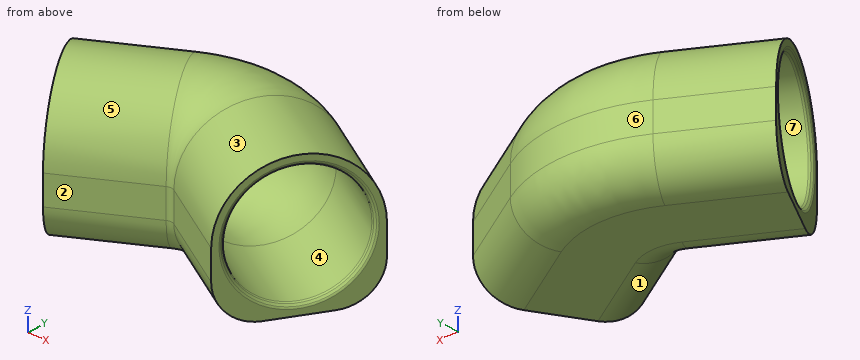
```python
from build123d import *

# Parameters (mm, degrees)
F1_R    = 11.1633
F3_R    = 7.62
F4_SIZE = 0.635
F5_R    = 0.508


with BuildPart() as f2:
    # F2: sweep along a path in F0
    with BuildLine(Plane.XY) as f2_path:
        Line((-21.9970452561, -12.7), (-6.35, -3.6661742094))
        ThreePointArc((-6.35, -3.6661742094), (0, -1.9646968374), (6.35, -3.6661742094))
        Line((6.35, -3.6661742094), (21.9970452561, -12.7))
    # F1 (on Right) → F2 (sweep)
    with BuildSketch(Plane.YZ):
        with BuildLine():
            ThreePointArc((0, -13.1633), (9.3078586928, -9.3078586928), (13.1633, 0))
            ThreePointArc((13.1633, 0), (0, 13.1633), (-13.1633, 0))
            ThreePointArc((-13.1633, 0), (-9.3078586928, -9.3078586928), (0, -13.1633))
        make_face()
        Circle(F1_R, mode=Mode.SUBTRACT)
        with BuildLine():
            Line((13.1633, -13.1633), (13.1633, 0))
            ThreePointArc((13.1633, 0), (9.3078586928, -9.3078586928), (0, -13.1633))
            Line((0, -13.1633), (13.1633, -13.1633))
        make_face()
        with BuildLine():
            ThreePointArc((0, -13.1633), (-9.3078586928, -9.3078586928), (-13.1633, 0))
            Line((-13.1633, 0), (-13.1633, -13.1633))
            Line((-13.1633, -13.1633), (0, -13.1633))
        make_face()
    sweep(path=f2_path.line)

    # F3
    f3_edges = [f2.edges().sort_by_distance(p)[0] for p in [
        (-8.574221, -17.881362, -13.1633),
        (8.574221, -17.881362, -13.1633),
        (0, -13.1633, -13.1633),
        (21.737521, 4.918142, -13.1633),
        (0, 13.1633, -13.1633),
        (-21.737521, 4.918142, -13.1633),
    ]]
    fillet(f3_edges, radius=F3_R)

    # F4
    f4_edges = [f2.edges().sort_by_distance(p)[0] for p in [
        (17.397744, -20.666224, 0),
        (-17.397744, -20.666224, 0),
    ]]
    chamfer(f4_edges, length=F4_SIZE)

    # F5
    f5_edges = [f2.edges().sort_by_distance(p)[0] for p in [
        (-17.080244, -21.21615, 0),
        (-16.847818, -20.348724, 0),
        (17.080244, -21.21615, 0),
        (16.847818, -20.348724, 0),
    ]]
    fillet(f5_edges, radius=F5_R)


solid = f2.part
```
Could you check a few things on this model? Use its own coordinates, in mm. Face numbers are marked on the shaded views. A direction names the side the tool comes from. Give positions to 0.01 mm unless a question says otherwise; leave off trailing zeros.
Q1. If I drill on line 1 along Z through (x, y) = (-6, -10.5); line 2 along X through (y, z) = (6, 4.5); line 3 along Z through (x, y) = (6, -4), over which ranges is the centre line in solid material (lowest first)?
Q2. I'm going to push flat-ended pins straight in: P1, Ø6, axis at y = 3.5, z = 8, coming from the -X side; P2, Ø2, axis at y = -0.5, z = -8.5, coming from the +X side; P3, Ø2, axis at y = -18, z = -8.5, coming from the -X side. Where does each tip first touch, or does it pass through?
Q3. We'd pull the mould along Y, two halves only. Please class the marked faces 4, 5, 6 and 7: +Y half, -Y half, draft (parallel to the pull), parting line (faces both ways), or undercut.
Q4. For the marked faces 1, 2 and 3, which set-ups out of +Z, -Z, +X, -X, +Y, -Y let a thin tool reach every point of the face, with its end or its side?
Solution:
1. line 1: z = -12.74 to -7.73, 7.73 to 10.41
1. line 2: x = -18.28 to -13.97, 13.97 to 18.28
1. line 3: z = -13.16 to -10.9, 10.9 to 12.94
2. P1: stops at x = -25.27
2. P2: stops at x = 29.4
2. P3: stops at x = -19.27
3. face 4: undercut
3. face 5: parting line
3. face 6: +Y half
3. face 7: undercut
4. face 1: -Z, -Y
4. face 2: +Z, -Z, -Y
4. face 3: +Z
